Input: dimensioned drawing with shaded views. Units: mm. Origin: part minimum x, y, z. Coordinates: 2 decimals unless noted, no trailing zeros. Loops run counter-clockwise (first coordinate to the right, second up) from the corner with the lowest first, then second, coordinate; pieces in that order, holes last.
Item 1: Section B-B on y = 74. Return loops of the section in (x, z) (1 decimal), and give its area (3 significant figures).
Item 2: Ray query, line 1 along Y through (x, z) = (5, 1.15) (1 decimal); line 2 along X through (y, z) = (74, 1.2) (1 decimal). Return the intervals inside material, ascending.
Item 3: Contact query for a flat-ended pin moving along its axis: P1, Ø2.5, axis at x = 105, y = 6, coming from the +Z side. Output: stop coordinate, or through.
Item 4: Section A-A on x = 5. Return loops of the section in (y, z) (1 decimal).
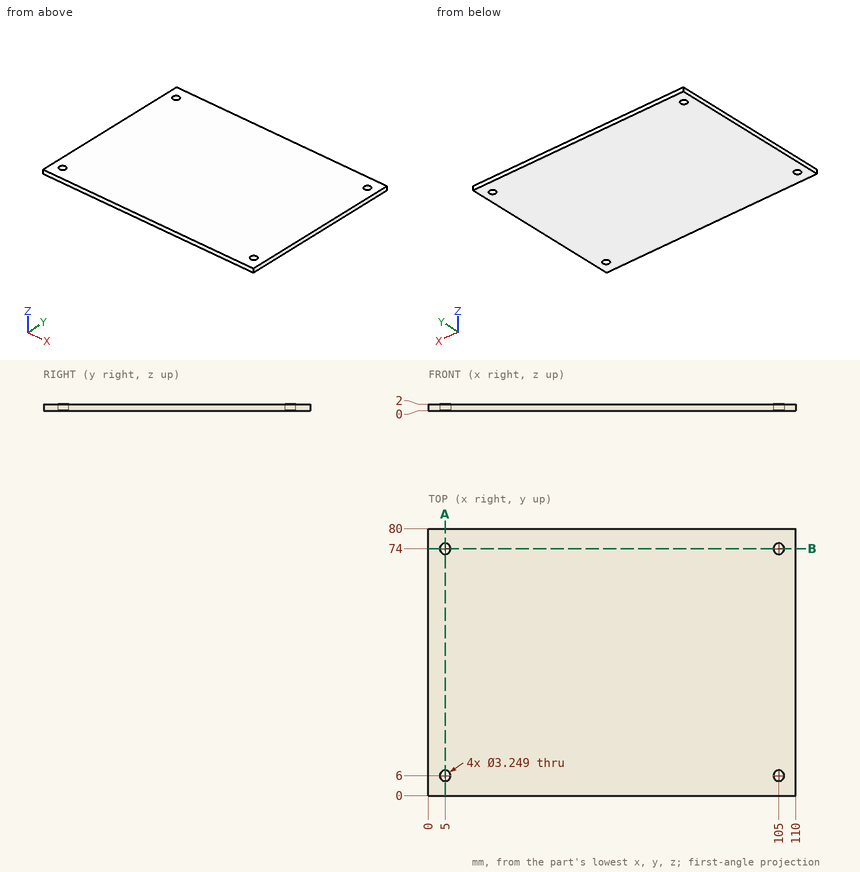
Results found:
1. outline: (0, 0) - (3.4, 0) - (3.4, 2) - (0, 2) - close; (6.6, 0) - (103.4, 0) - (103.4, 2) - (6.6, 2) - close; (106.6, 0) - (110, 0) - (110, 2) - (106.6, 2) - close
1. area: 207 mm2
2. line 1: y = 0 to 4.4, 7.6 to 72.4, 75.6 to 80
2. line 2: x = 0 to 3.4, 6.6 to 103.4, 106.6 to 110
3. P1: passes through
4. outline: (0, 0) - (4.4, 0) - (4.4, 2) - (0, 2) - close; (7.6, 0) - (72.4, 0) - (72.4, 2) - (7.6, 2) - close; (75.6, 0) - (80, 0) - (80, 2) - (75.6, 2) - close
